Check sheet for the modelled part. Datum: model origin and axes. Units: mm. A direction names the side the tool comes from. Round coordinates to 2 decimals unless told otherwise and drop trailing zeros. Loops run counter-clockwise (first coordinate to the right, second up) from the corner with the lowest first, then second, coordinate; pieces in that order, holes last. Notation, with made-up numbers: (76, -2.5) - (105, -2.5) arc R9 ccw to (105, 5.5) - close; hole circle Ø10 at (25.5, 73). An arc over 180 degrees is marked (long way). Put each result on its own line as item: value. Start each with the question number.
```python
from build123d import *

# Parameters (mm, degrees)
SKETCH_1_R          = 11.15
SKETCH_1_R_2        = 1.5
SKETCH_1_R_3        = 2.5
EXTRUDE_1_DEPTH     = 34
SKETCH_1_3_R        = 1.5
CUT_EXTRUDE_1_DEPTH = 4.5
SKETCH_1_4_R        = 11.15
SKETCH_1_4_R_2      = 2.5
EXTRUDE_2_DEPTH     = 2
SKETCH_1_5_R        = 2.5
EXTRUDE_3_DEPTH     = 24
CHAMFER_1_SIZE      = 0.5
CUT_EXTRUDE_2_DEPTH = 23


with BuildPart() as part:
    # Sketch 1 → Extrude 1 (new body)
    # profile 1 of 7: a face of its own
    with BuildSketch(Plane(origin=(0, 0, 0), x_dir=(1, 0, 0), z_dir=(0, 1, 0))):
        Polygon((-21.15, -16.15), (-21.15, 16.15), (-16.15, 21.15), (16.15, 21.15), (21.15, 16.15), (21.15, -16.15), (16.15, -21.15), (-16.15, -21.15), align=None)
        Circle(SKETCH_1_R, mode=Mode.SUBTRACT)
        with Locations((15.5, 15.5)):
            Circle(SKETCH_1_R_2, mode=Mode.SUBTRACT)
        with Locations((-15.5, 15.5)):
            Circle(SKETCH_1_R_2, mode=Mode.SUBTRACT)
        with Locations((15.5, -15.5)):
            Circle(SKETCH_1_R_2, mode=Mode.SUBTRACT)
        with Locations((-15.5, -15.5)):
            Circle(SKETCH_1_R_2, mode=Mode.SUBTRACT)
    # profile 2 of 7: a face of its own
    with BuildSketch(Plane(origin=(0, 0, 0), x_dir=(1, 0, 0), z_dir=(0, 1, 0))):
        with Locations((-15.5, 15.5)):
            Circle(SKETCH_1_R_2)
    # profile 3 of 7: a face of its own
    with BuildSketch(Plane(origin=(0, 0, 0), x_dir=(1, 0, 0), z_dir=(0, 1, 0))):
        with Locations((-15.5, -15.5)):
            Circle(SKETCH_1_R_2)
    # profile 4 of 7: a face of its own
    with BuildSketch(Plane(origin=(0, 0, 0), x_dir=(1, 0, 0), z_dir=(0, 1, 0))):
        Circle(SKETCH_1_R)
        Circle(SKETCH_1_R_3, mode=Mode.SUBTRACT)
    # profile 5 of 7: a face of its own
    with BuildSketch(Plane(origin=(0, 0, 0), x_dir=(1, 0, 0), z_dir=(0, 1, 0))):
        Circle(SKETCH_1_R_3)
    # profile 6 of 7: a face of its own
    with BuildSketch(Plane(origin=(0, 0, 0), x_dir=(1, 0, 0), z_dir=(0, 1, 0))):
        with Locations((15.5, -15.5)):
            Circle(SKETCH_1_R_2)
    # profile 7 of 7: a face of its own
    with BuildSketch(Plane(origin=(0, 0, 0), x_dir=(1, 0, 0), z_dir=(0, 1, 0))):
        with Locations((15.5, 15.5)):
            Circle(SKETCH_1_R_2)
    extrude(amount=-EXTRUDE_1_DEPTH)

    # Sketch 1_3 → Cut-Extrude 1 (cut)
    with BuildSketch(Plane(origin=(0, 0, 0), x_dir=(1, 0, 0), z_dir=(0, 1, 0))):
        with Locations(Location((-15.5, 15.5, 0), (0, 0, 270))):
            Circle(SKETCH_1_3_R)
        with Locations(Location((-15.5, -15.5, 0), (0, 0, 270))):
            Circle(SKETCH_1_3_R)
        with Locations(Location((15.5, 15.5, 0), (0, 0, 270))):
            Circle(SKETCH_1_3_R)
        with Locations(Location((15.5, -15.5, 0), (0, 0, 270))):
            Circle(SKETCH_1_3_R)
    extrude(amount=-CUT_EXTRUDE_1_DEPTH, mode=Mode.SUBTRACT)

    # Sketch 1_4 → Extrude 2 (add)
    with BuildSketch(Plane(origin=(0, 0, 0), x_dir=(1, 0, 0), z_dir=(0, 1, 0))):
        with Locations(Location((0, 0, 0), (0, 0, 270))):
            Circle(SKETCH_1_4_R)
        with Locations(Location((0, 0, 0), (0, 0, 270))):
            Circle(SKETCH_1_4_R_2, mode=Mode.SUBTRACT)
    extrude(amount=EXTRUDE_2_DEPTH)

    # Sketch 1_5 → Extrude 3 (add)
    with BuildSketch(Plane(origin=(0, 0, 0), x_dir=(1, 0, 0), z_dir=(0, 1, 0))):
        with Locations(Location((0, 0, 0), (0, 0, 270))):
            Circle(SKETCH_1_5_R)
    extrude(amount=EXTRUDE_3_DEPTH)

    # Chamfer 1
    chamfer_1_edges = [part.edges().sort_by_distance(p)[0] for p in [
        (21.15, 0, 0),
        (18.65, 0, 18.65),
        (0, 0, 21.15),
        (-18.65, 0, 18.65),
        (-21.15, 0, 0),
        (-15.5, 0, -17),
        (-15.5, 0, 14),
        (15.5, 0, -17),
        (15.5, 0, 14),
        (0, 2, -2.5),
        (0, 0, -11.15),
        (0, 2, -11.15),
        (0, 24, -2.5),
        (-18.65, 0, -18.65),
        (0, 0, -21.15),
        (18.65, 0, -18.65),
    ]]
    chamfer(chamfer_1_edges, length=CHAMFER_1_SIZE)

    # Sketch 2 → Cut-Extrude 2 (cut)
    with BuildSketch(Plane(origin=(0, -29, 0), x_dir=(-1, 0, 0), z_dir=(0, -1, 0))):
        Polygon((21.15, -16.15), (21.15, 16.15), (16.15, 21.15), (-16.15, 21.15), (-21.15, 16.15), (-21.15, -16.15), (-16.15, -21.15), (16.15, -21.15), align=None)
        Polygon((20.15, -15.735786438), (20.15, 15.735786438), (15.735786438, 20.15), (-15.735786438, 20.15), (-20.15, 15.735786438), (-20.15, -15.735786438), (-15.735786438, -20.15), (15.735786438, -20.15), align=None, mode=Mode.SUBTRACT)
    extrude(amount=-CUT_EXTRUDE_2_DEPTH, mode=Mode.SUBTRACT)


solid = part.part
```
Q1. Cross-section at D-D on y = -30. Enter the section's corners in (x, z), and give its area (3 significant figures).
Q2. Depth check by flat-ended pin: pin 1 Ø2 at (y, z) = (-11.5, -13.5) entering from +X; pin 2 Ø0.9 at (x, z) = (16, -15) entering from +Y; pin 3 Ø2.5 at (x, z) = (-15.5, -16) entering from +Y. Enter the tip coordinate at first touch or a pass-through.
Q3. Draft check along Z on faces 1 (the face through (-18.44, -0.25, 18.51)), 2 (the face through (20.5, -29, -0.1)), 3 (the face through (15.57, -2.47, -17)), 4 (the face through (-17.974, -17.661, -17.912)). Enter one of: +Z half, -Z half, draft (parallel to the pull), parting line (faces both ways), or undercut.
Q4. Cross-section at B-B on y = -21.5. Enter the section's corners in (x, z), and give its area (3 significant figures).
Q5. Material ranges on line 1 (X direction, y = -2, z = 15.5); line 2 (Y direction, x = -2, z = -5.5); line 3 (Y direction, x = 16, z = 3.5), recorded low to high. Write a range as from..to.
Q6. Set-up check for faces 5 (the face through (17.974, -17.661, 17.912)), 6 (the face through (-15, -4.5, 15)), 7 (the face through (20.5, -6, -0.1)), 8 (the face through (0, -18, 20.15)): record each of +Z, -Z, +X, -X, +Y, -Y from which the full face is reachable in a straight line by a thin tool's end or side.
Answer list:
1. outline: (-21.15, -16.15) - (-16.15, -21.15) - (16.15, -21.15) - (21.15, -16.15) - (21.15, 16.15) - (16.15, 21.15) - (-16.15, 21.15) - (-21.15, 16.15) - close
1. area: 1,740 mm2
2. pin 1: stops at x = 20.15
2. pin 2: stops at y = -4.5
2. pin 3: stops at y = -0.25
3. face 1: +Z half
3. face 2: draft
3. face 3: undercut
3. face 4: -Z half
4. outline: (-20.15, -15.74) - (-15.74, -20.15) - (15.74, -20.15) - (20.15, -15.74) - (20.15, 15.74) - (15.74, 20.15) - (-15.74, 20.15) - (-20.15, 15.74) - close
4. area: 1,590 mm2
5. line 1: x = -21.15..-17, -14..14, 17..21.15
5. line 2: y = -34..2
5. line 3: y = -34..0
6. face 5: +Z, +X
6. face 6: +Y
6. face 7: none
6. face 8: +Z, +X, -X
